Verification items for this drawing (mm, ordinates from the low corner). A direction names the side the tool comes from. Round coordinates to 2 decimals unless told otherwise and drop trailing zeros. Order: outer loops, then holes, each group sorted by start corner. A loop starts at its lowest first (then second) coordinate and runs counter-clockwise, first axis right, second up. Notation, with made-up numbers: M 68.25,76.25 L 73.25,76.25 A24 ccw 73.25,99.25 Z; hole C 60,-5.5 d3. An arc over 180 degrees is marked long. Return JSON: item names as keys, results as strings. Group by question number.
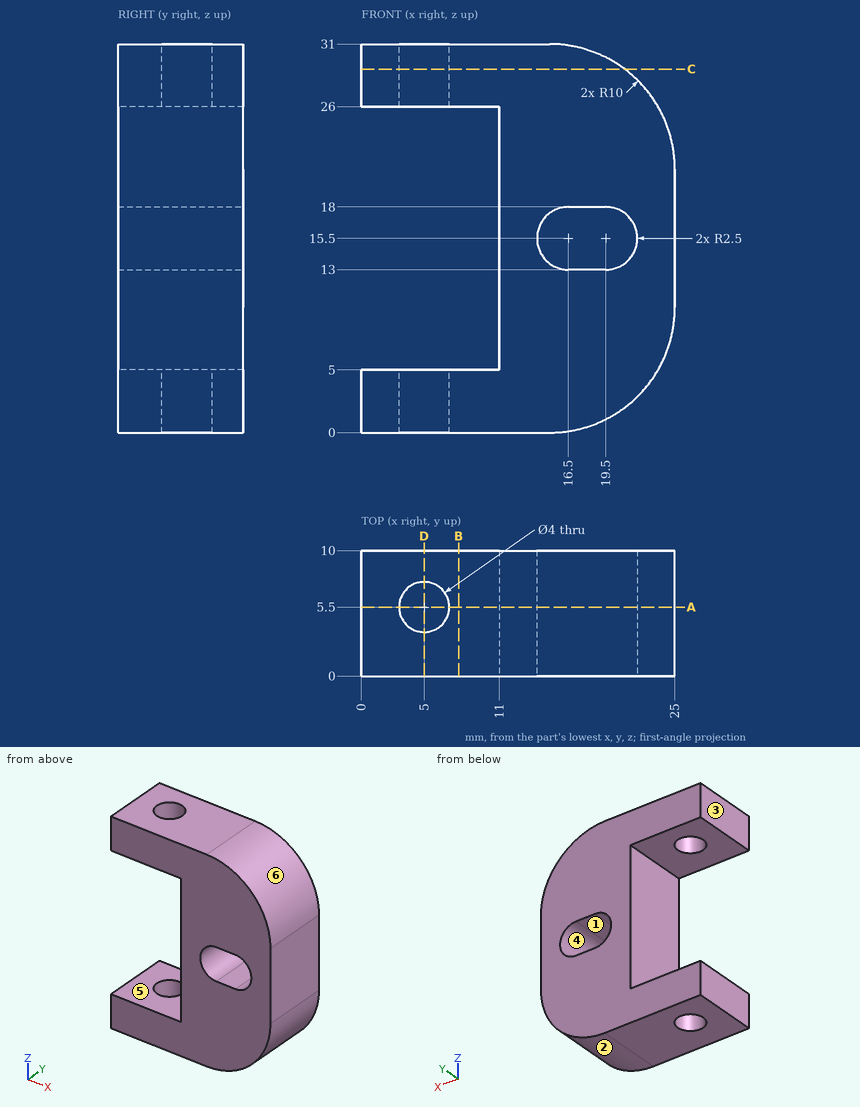
1. Thickness scan on line 1 along Z through (x, y) = (8.5, 3.5); line 2 along Y through (x, z) = (5, 1.7); line 3 along X through (y, z) = (5.25, 16). Record the ranges inside material, lowest first. Write a range as from..to.
2. Access from +Z, -Z, +X, -X, +Y, -Y to the whole of each face (thin tool, end or side, straight path). Record for the marked faces 4, 5 and 6.
3. Cross-section at D-D (x = 5). Enter the section's corners in (y, z).
4. Cross-section at C-C (z = 29). Enter the section's corners in (x, y).
5. Draft check along X on the marked faces 1, 2 and 3. Enter one of: +X half, -X half, draft (parallel to the pull), parting line (faces both ways), or undercut.
6. Cross-section at A-A (y = 5.5). Enter the section's corners in (x, z).
7. Go/stop test with flat-tipped pins: pin 1 (5 mm diameter, centred on x = 21, y = 4.5, fed in from -Z); pin 2 (2.5 mm diameter, centred on x = 18, y = 7, fed in from +Z); pin 3 (3.5 mm diameter, centred on x = 17.5, y = 4.5, fed in from -Z); pin 4 (3.5 mm diameter, centred on x = 5, y = 5.5, fed in from +Z). Record where each tip stops, or that it passes through.
8. Cross-section at B-B (x = 7.75). Enter the section's corners in (y, z).
Computed:
{
 "1": {"line 1": "z = 0..5, 26..31", "line 2": "y = 0..3.5, 7.5..10", "line 3": "x = 11..14.05, 21.95..25"},
 "2": {"face 4": "+Y, -Y", "face 5": "-X, +Y, -Y", "face 6": "+Z, +X, +Y, -Y"},
 "3": {"outline": "M 0,0 L 3.5,0 L 3.5,5 L 0,5 Z; M 0,26 L 3.5,26 L 3.5,31 L 0,31 Z; M 7.5,0 L 10,0 L 10,5 L 7.5,5 Z; M 7.5,26 L 10,26 L 10,31 L 7.5,31 Z"},
 "4": {"outline": "M 0,0 L 21,0 L 21,10 L 0,10 Z; hole C 5,5.5 d4"},
 "5": {"face 1": "undercut", "face 2": "+X half", "face 3": "-X half"},
 "6": {"outline": "M 0,0 L 3,0 L 3,5 L 0,5 Z; M 0,26 L 3,26 L 3,31 L 0,31 Z; M 7,0 L 15,0 A10 ccw 25,10 L 25,21 A10 ccw 15,31 L 7,31 L 7,26 L 11,26 L 11,5 L 7,5 Z; hole M 16.5,13 L 19.5,13 A2.5 ccw 19.5,18 L 16.5,18 A2.5 ccw Z"},
 "7": {"pin 1": "stops at z = 0.63", "pin 2": "stops at z = 30.85", "pin 3": "stops at z = 0.03", "pin 4": "passes through"},
 "8": {"outline": "M 0,0 L 10,0 L 10,5 L 0,5 Z; M 0,26 L 10,26 L 10,31 L 0,31 Z"}
}
